Geometry: see drawing. Coordinates: mm, zero at the bounding-box minimum. A direction names the side the tool comes from. Round coordinates to 2 decimals unless told otherwise and drop trailing zeros. Loops run counter-clockwise (first coordinate to the right, second up) from the corner with the lowest first, then second, coordinate; pieces in that order, holes last. Notation, with made-up numbers: (-17.75, 8) - (-6.75, 8) arc R18 cw to (-6.75, 25) - close; hole circle Ø3 at (-24.75, 3.5). An arc over 180 degrees is marked (long way). Use CSV: the item, a comma, the result in double quotes. Start each with the question number.
1. Material intervals for probe 1 along Y at (x, z) = (11.5, 3.25) (1 decimal); probe 2 along X at (y, z) = (38, 19.75); probe 3 along Z at (x, y) = (9, 42), sorted ascending. Write a range as from..to.
2. Pull-direction query (X, two-part tool) for the marked faces 5, 6 and 7; classes: +X half, -X half, draft (parallel to the pull), parting line (faces both ways), or undercut.
3. Cut plane A-A (x = 31.75). Return loops of the section in (y, z) (1 decimal).
4. Access query for the marked faces 1, 2, 3 and 4. Directions: +Z, -Z, +X, -X, +Y, -Y. A direction counts if a zero-diameter tool reaches every point of the face in a straight line with its end or side. Return the directions, or none.
5. Pin query (flat end, axial travel): P1, Ø3, axis at x = 50.5, y = 54.5, coming from the +Z side; P2, Ø9, axis at x = 14, y = 13, coming from the +Z side; P3, Ø9.5, axis at x = 26, z = 22.5, coming from the -Y side (3 decimals). Return the tip coordinate at first contact, or that it passes through.
6. Cut plane C-C (y = 51.5). Return loops of the section in (x, z) (1 decimal), and give its area (3 significant figures).
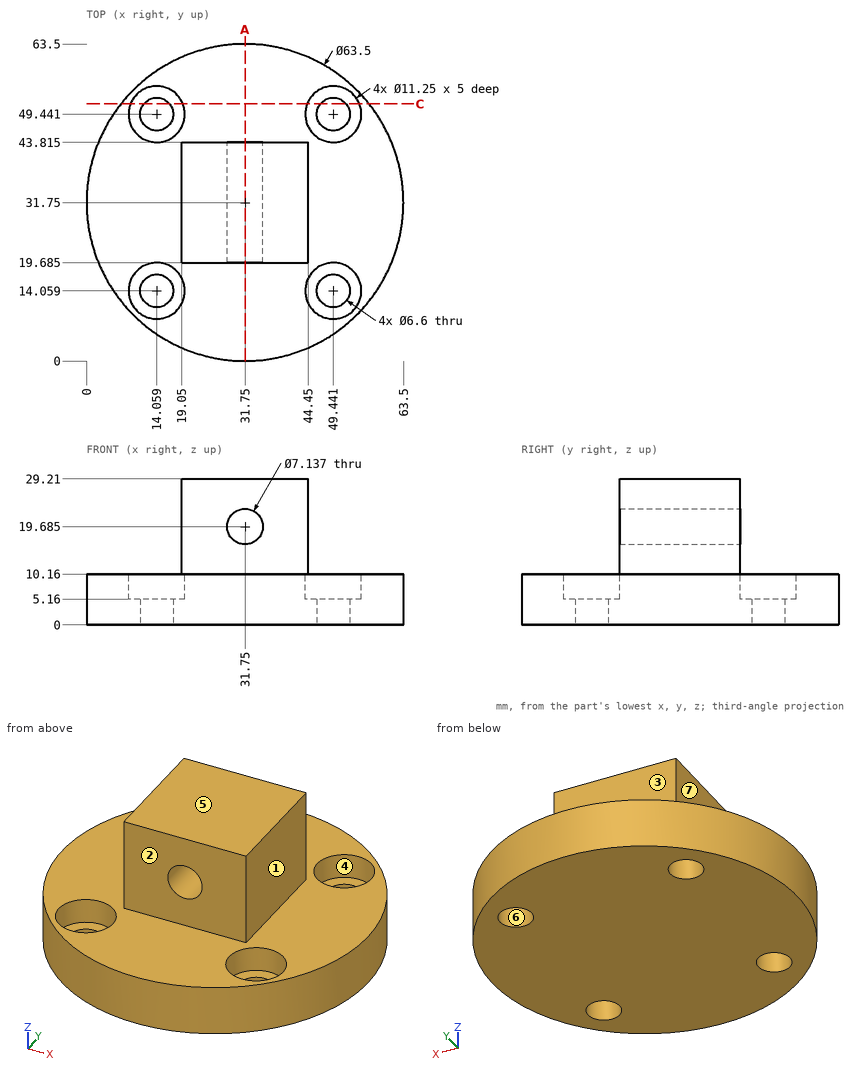
Established:
1,probe 1,"y = 7.3..12, 16.1..47.4, 51.5..56.2"
1,probe 2,"x = 19.05..28.18, 35.32..44.45"
1,probe 3,"z = 0..10.16"
2,face 5,"draft"
2,face 6,"undercut"
2,face 7,"-X half"
3,outline,"(0, 0) - (63.5, 0) - (63.5, 10.2) - (43.8, 10.2) - (43.8, 16.1) - (19.7, 16.1) - (19.7, 10.2) - (0, 10.2) - close; (19.7, 23.3) - (43.8, 23.3) - (43.8, 29.2) - (19.7, 29.2) - close"
4,face 1,"+Z, +X, +Y, -Y"
4,face 2,"+Z, +X, -X, -Y"
4,face 3,"+Z, +X, -X, +Y"
4,face 4,"+Z"
5,P1,"stops at z = 10.16"
5,P2,"stops at z = 5.16"
5,P3,"stops at y = 19.685"
6,outline,"(6.9, 0) - (11.5, 0) - (11.5, 5.2) - (8.8, 5.2) - (8.8, 10.2) - (6.9, 10.2) - close; (16.6, 0) - (46.9, 0) - (46.9, 5.2) - (44.2, 5.2) - (44.2, 10.2) - (19.3, 10.2) - (19.3, 5.2) - (16.6, 5.2) - close; (52, 0) - (56.6, 0) - (56.6, 10.2) - (54.7, 10.2) - (54.7, 5.2) - (52, 5.2) - close"
6,area,"347 mm2"
